```python
from build123d import *

# Parameters (mm, degrees)
SKETCH2_W             = 190
SKETCH2_H             = 190
EXTRUDE1_DEPTH        = 10
SKETCH3_R             = 19
SKETCH3_R_2           = 4
EXTRUDE2_DEPTH        = 10
FILLET1_R             = 30
M8_TAPPED_HOLE1_D     = 6.8
M8_TAPPED_HOLE1_DEPTH = 19.75
M8_TAPPED_HOLE1_TIP   = 2.042926105


with BuildPart() as part:
    # Sketch2 → Extrude1 (new body)
    with BuildSketch(Plane(origin=(0, 0, 0), x_dir=(1, 0, 0), z_dir=(0, 1, 0))):
        Rectangle(SKETCH2_W, SKETCH2_H)
    extrude(amount=EXTRUDE1_DEPTH)

    # Sketch3 → Extrude2 (cut)
    with BuildSketch(Plane(origin=(0, 10, 0), x_dir=(1, 0, 0), z_dir=(0, 1, 0))):
        with Locations(Location((0, 0, 0), (0, 0, 270))):
            Circle(SKETCH3_R)
        with Locations(Location((-75, 75, 0), (0, 0, 270))):
            Circle(SKETCH3_R_2)
        with Locations(Location((75, 75, 0), (0, 0, 90))):
            Circle(SKETCH3_R_2)
        with Locations(Location((75, -75, 0), (0, 0, 270))):
            Circle(SKETCH3_R_2)
        with Locations(Location((-75, -75, 0), (0, 0, 90))):
            Circle(SKETCH3_R_2)
    extrude(amount=-EXTRUDE2_DEPTH, mode=Mode.SUBTRACT)

    # Fillet1
    fillet1_edges = [part.edges().sort_by_distance(p)[0] for p in [
        (-95, 5, -95),
        (95, 5, -95),
        (95, 5, 95),
        (-95, 5, 95),
    ]]
    fillet(fillet1_edges, radius=FILLET1_R)

    # M8 Tapped Hole1
    with Locations(Plane(origin=(-24.748737342, 10, -24.748737342), x_dir=(0, 0, 1), z_dir=(0, 1, 0))):
        with Locations((0, 0), (0, 49.497474684), (49.497474684, 0), (49.497474684, 49.497474684)):
            Hole(M8_TAPPED_HOLE1_D / 2, depth=M8_TAPPED_HOLE1_DEPTH)
            with Locations((0, 0, -(M8_TAPPED_HOLE1_DEPTH + M8_TAPPED_HOLE1_TIP / 2))):  # 118° drill point
                Cone(0, M8_TAPPED_HOLE1_D / 2, M8_TAPPED_HOLE1_TIP, mode=Mode.SUBTRACT)


solid = part.part
```
Verification items for the finished model (mm, model axes). Coordinates: 2 decimals unless noted, no trailing zeros. Order: outer loops, then holes, each group sorted by start corner. A loop starts at its lowest first (then second) coordinate and runs counter-clockwise, first axis right, second up. Notation, with made-up numbers: (18, 72.5) -> (42, 72.5) arc R15 cw to (42, 92.5) -> close; hole circle Ø4 at (67.5, 85.5). An arc over 180 degrees is marked (long way). Answer as CSV lines item,"result". Start each with the question number.
1) Release check for a two-part mould opening along X. For faces 1 (the face through (-86.445, 5.07, -85.979)), 2 (the face through (-23.727, 4.93, 21.506)), 3 (the face through (85.979, 5.07, -86.445)) record: released by +X, released by -X, zero draft, split by the parting line, or undercut.
2) Cross-section at C-C, the plane z = -75. Record the boundary of the cut face in (x, y), then the cut area to 3 significant figures.
3) Gauge pin test, flat end, axial feed: pin 1 Ø7 at (x, z) = (75, 75) entering from +Y. Record the tip position at first contact, or that the pin passes through.
4) Cross-section at D-D, the plane y = 6.75. Give the number of separate pieces and of enclosed holes in the cut face, then the cut area to 3 significant figures.
5) Material ranges on L1, parallel to X at y = 7.75, z = -24; L2, parallel to X at y = 6.75, z = 0; L3, parallel to X at y = 4.5, z = -75, recorded low to high. Write a range as [from, to].
6) Cross-section at B-B, the plane z = 0. Record the boundary of the cut face in (x, y).
7) Cross-section at A-A, the plane x = 0. Record the boundary of the cut face in (y, z).
Conclusion:
1,face 1,"released by -X"
1,face 2,"undercut"
1,face 3,"released by +X"
2,outline,"(-93.28, 0) -> (-79, 0) -> (-79, 10) -> (-93.28, 10) -> close; (-71, 0) -> (71, 0) -> (71, 10) -> (-71, 10) -> close; (79, 0) -> (93.28, 0) -> (93.28, 10) -> (79, 10) -> close"
2,area,"1,710 mm²"
3,pin 1,"passes through"
4,separate pieces,"1"
4,enclosed holes,"9"
4,area,"33,800 mm²"
5,L1,"x = [-95, -28.07], [-21.43, 21.43], [28.07, 95]"
5,L2,"x = [-95, -19], [19, 95]"
5,L3,"x = [-93.28, -79], [-71, 71], [79, 93.28]"
6,outline,"(-95, 0) -> (-19, 0) -> (-19, 10) -> (-95, 10) -> close; (19, 0) -> (95, 0) -> (95, 10) -> (19, 10) -> close"
7,outline,"(0, -95) -> (10, -95) -> (10, -19) -> (0, -19) -> close; (0, 19) -> (10, 19) -> (10, 95) -> (0, 95) -> close"
